Verification items for this drawing (mm, ordinates from the low corner). A direction names the side the tool comes from. Round coordinates to 2 decimals unless told otherwise and drop trailing zeros. Loops run counter-clockwise (first coordinate to the right, second up) from the corner with the lowest first, then second, coordinate; pieces in that order, holes last. Notation, with made-up numbers: (84.25, 71) - (109.25, 71) arc R20 cw to (109.25, 92) - close; hole circle Ø1 at (50.25, 61.25). An arc over 180 degrees is marked (long way). Answer in a Markdown table with one row per item. Add a question column.
(1) Cross-section at B-B on z = 23. Enter the section's corners in (x, y), then the cut area to 3 significant figures.
(2) Access from +Z, -Z, +X, -X, +Y, -Y to the whole of each face (thin tool, end or side, straight path). Record for the marked faces 5, 6 and 7.
(3) Cross-section at C-C on y = 42.5. Enter the section's corners in (x, z), then the cut area to 3 significant figures.
(4) Mould release check, pull along X, two halves, no side actions. Record for the marked faces 1, 2, 3 and 4: +X half, -X half, draft (parallel to the pull), parting line (faces both ways), or undercut.
(5) Cross-section at D-D on y = 32.5. Enter the section's corners in (x, z).
(6) Cross-section at A-A on x = 20. Enter the section's corners in (y, z) (1 decimal), then the cut area to 3 significant figures.
(7) Gauge pin test, flat ends, axial feed: pin 1 (13.5 mm diameter, centred on y = 31, z = 34, fed in from +X); pin 2 (1 mm diameter, centred on y = 11, z = 12.5, fed in from +X); pin 3 (4 mm diameter, centred on x = 12, y = 26, fed in from -Z); pin 4 (3 mm diameter, centred on x = 29.5, y = 51.5, fed in from +Z). Record the tip position at first contact, or that the pin passes through.
(8) Thickness scan on line 1 along Z through (x, y) = (17.5, 57.5) (1 decimal); line 2 along X through (y, z) = (59, 40.5); line 3 along Z through (x, y) = (23, 39). Record the ranges inside material, lowest first.
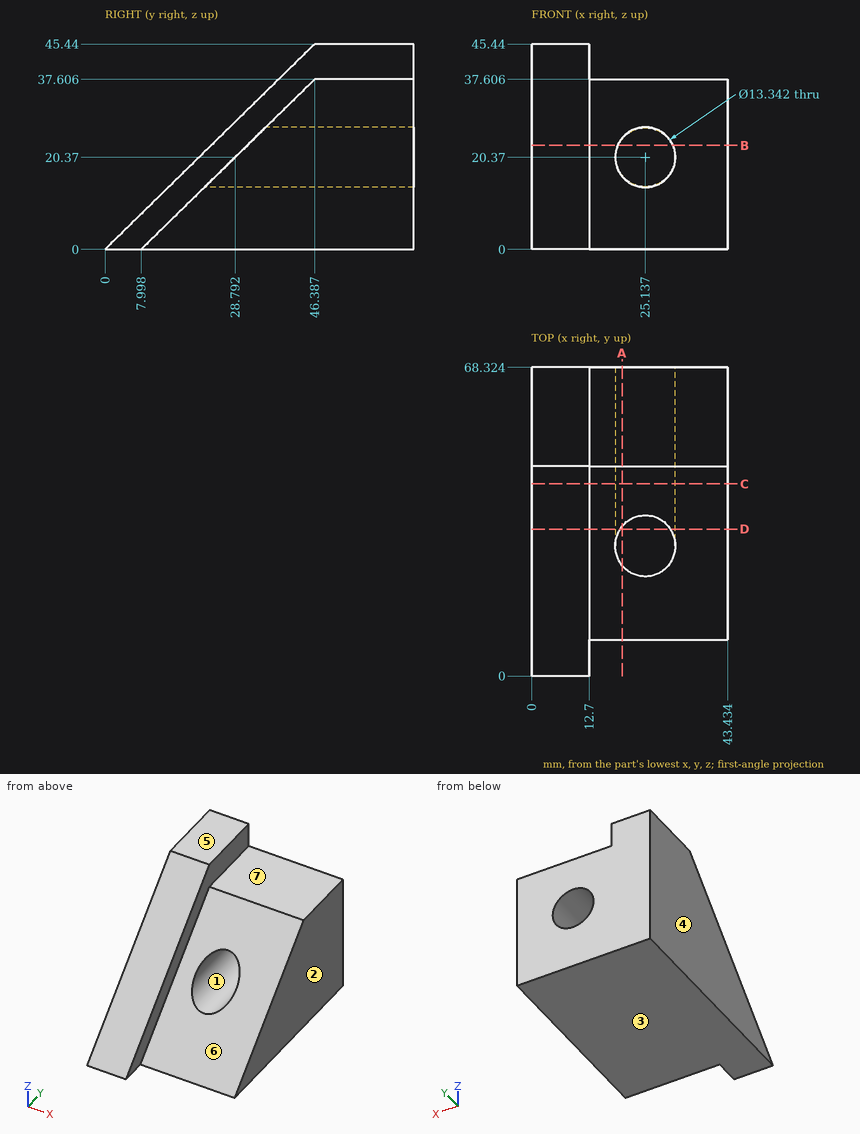
Answers:
| question | item | result |
|---|---|---|
| 1 | outline | (0, 23.48) - (12.7, 23.48) - (12.7, 31.48) - (19.01, 31.48) - (19.01, 68.32) - (0, 68.32) - close; (31.27, 31.48) - (43.43, 31.48) - (43.43, 68.32) - (31.27, 68.32) - close |
| 1 | area | 1,250 mm^2 |
| 2 | face 5 | +Z, +X, -X, +Y, -Y |
| 2 | face 6 | +Z, +X, -Y |
| 2 | face 7 | +Z, +X, +Y, -Y |
| 3 | outline | (0, 0) - (43.43, 0) - (43.43, 33.8) - (12.7, 33.8) - (12.7, 41.63) - (0, 41.63) - close; hole circle Ø13.34 at (25.14, 20.37) |
| 3 | area | 1,430 mm^2 |
| 4 | face 1 | undercut |
| 4 | face 2 | +X half |
| 4 | face 3 | draft |
| 4 | face 4 | -X half |
| 5 | outline | (0, 0) - (43.43, 0) - (43.43, 24) - (30.73, 24) arc R6.67 cw (long way) to (19.54, 24) - (12.7, 24) - (12.7, 31.84) - (0, 31.84) - close |
| 6 | outline | (8, 0) - (68.3, 0) - (68.3, 16.1) - (24.4, 16.1) - close; (33.1, 24.6) - (68.3, 24.6) - (68.3, 37.6) - (46.4, 37.6) - close |
| 6 | area | 1,210 mm^2 |
| 7 | pin 1 | stops at x = 12.7 |
| 7 | pin 2 | passes through |
| 7 | pin 3 | stops at z = 0 |
| 7 | pin 4 | stops at z = 37.61 |
| 8 | line 1 | z = 0 to 37.6 |
| 8 | line 2 | x = 0 to 12.7 |
| 8 | line 3 | z = 0 to 14.05, 26.69 to 30.37 |
